Part model, mm, in its own coordinate system. Face numbers are marked on the shaded views. A direction names the side the tool comes from. Give positions to 0.01 mm unless a question says otherwise; leave off trailing zeros. Order: outer loops, then holes, each group sorted by start corner. A loop starts at its lowest first (then second) coordinate and runs counter-clockwise, first axis right, second up.
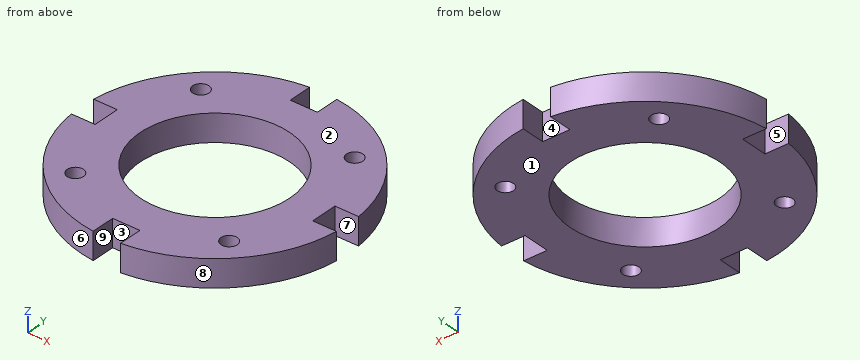
from build123d import *

# Parameters (mm, degrees)
ESQUISSE1_R        = 13.7
ESQUISSE1_R_2      = 1.5
BOSS_EXTRU_1_DEPTH = 5


with BuildPart() as part:
    # Esquisse1 → Boss.-Extru.1 (new body)
    with BuildSketch(Plane.XY):
        with BuildLine():
            Line((24.372115214, 2.5), (20, 2.5))
            Line((20, 2.5), (20, -2.5))
            Line((20, -2.5), (24.372115214, -2.5))
            ThreePointArc((24.372115214, -2.5), (17.324116139, -17.324116139), (2.5, -24.372115214))
            Line((2.5, -24.372115214), (2.5, -20))
            Line((2.5, -20), (-2.5, -20))
            Line((-2.5, -20), (-2.5, -24.372115214))
            ThreePointArc((-2.5, -24.372115214), (-17.324116139, -17.324116139), (-24.372115214, -2.5))
            Line((-24.372115214, -2.5), (-20, -2.5))
            Line((-20, -2.5), (-20, 2.5))
            Line((-20, 2.5), (-24.372115214, 2.5))
            ThreePointArc((-24.372115214, 2.5), (-17.324116139, 17.324116139), (-2.5, 24.372115214))
            Line((-2.5, 24.372115214), (-2.5, 20))
            Line((-2.5, 20), (2.5, 20))
            Line((2.5, 20), (2.5, 24.372115214))
            ThreePointArc((2.5, 24.372115214), (17.324116139, 17.324116139), (24.372115214, 2.5))
        make_face()
        Circle(ESQUISSE1_R, mode=Mode.SUBTRACT)
        with Locations((14.142135624, 14.142135624)):
            Circle(ESQUISSE1_R_2, mode=Mode.SUBTRACT)
        with Locations(Location((14.142135624, -14.142135624, 0), (0, 0, 180))):
            Circle(ESQUISSE1_R_2, mode=Mode.SUBTRACT)
        with Locations(Location((-14.142135624, 14.142135624, 0), (0, 0, 180))):
            Circle(ESQUISSE1_R_2, mode=Mode.SUBTRACT)
        with Locations((-14.142135624, -14.142135624)):
            Circle(ESQUISSE1_R_2, mode=Mode.SUBTRACT)
    extrude(amount=BOSS_EXTRU_1_DEPTH)


solid = part.part
Item 1: Which spindle directions (+Z, -Z, +X, -X, +Y, -Y) get a long thin tool onto all of the face, cutting with end or side? Do the marked faces 1, 2, 3, 4 and 5. Say none if no direction does.
Item 2: Pull direction X, two halves, no side cores. Call the marked faces 6, 7, 8 and 9: released by +X, released by -X, zero draft, split by the parting line, or undercut.
Item 3: Band-saw the part on A-A on y = 0. List the corners of the cut face in (x, z), plus the area to 3 significant figures.
Item 4: Drill centre lines: probe 1 along Y at (x, z) = (0, 3.15); probe 2 along X at (y, z) = (2, 0.7); probe 3 along Y at (x, z) = (10.5, 3.6). Where is each one in solid material? Low to high.
Item 5: Drop flat-ended pins along their axis: P1, Ø1.5, axis at y = -1, z = 1.5, coming from the -X side; P2, Ø2, axis at x = -15.5, z = 0.5, coming from the -Y side; P3, Ø1.3, axis at y = 22.5, z = 1.5, coming from the +X side; P4, Ø2.5, axis at x = 14.14, y = -14.14, coming from the -Z side. Give the stop position or say it passes through.
Item 6: Band-saw the part on C-C on z = 1.2. List the corners of the cut face in (x, y).
Working result:
1. face 1: -Z, +X, -X, +Y, -Y
1. face 2: +Z, +X, -X, +Y, -Y
1. face 3: +Z, -Z, -Y
1. face 4: +Z, -Z, +Y
1. face 5: +Z, -Z, -X
2. face 6: released by -X
2. face 7: zero draft
2. face 8: released by +X
2. face 9: undercut
3. outline: (-20, 0) - (-13.7, 0) - (-13.7, 5) - (-20, 5) - close; (13.7, 0) - (20, 0) - (20, 5) - (13.7, 5) - close
3. area: 63.0 mm2
4. probe 1: y = -20 to -13.7, 13.7 to 20
4. probe 2: x = -20 to -13.55, 13.55 to 20
4. probe 3: y = -22.14 to -8.8, 8.8 to 22.14
5. P1: stops at x = -20
5. P2: stops at y = -19.75
5. P3: stops at x = 11.08
5. P4: passes through
6. outline: (-24.37, -2.5) arc R24.5 ccw to (-2.5, -24.37) - (-2.5, -20) - (2.5, -20) - (2.5, -24.37) arc R24.5 ccw to (24.37, -2.5) - (20, -2.5) - (20, 2.5) - (24.37, 2.5) arc R24.5 ccw to (2.5, 24.37) - (2.5, 20) - (-2.5, 20) - (-2.5, 24.37) arc R24.5 ccw to (-24.37, 2.5) - (-20, 2.5) - (-20, -2.5) - close; hole circle Ø3 at (-14.14, -14.14); hole circle Ø3 at (-14.14, 14.14); hole circle Ø27.4 at (0, 0); hole circle Ø3 at (14.14, -14.14); hole circle Ø3 at (14.14, 14.14)
